```python
from build123d import *

# Parameters (mm, degrees)
BOSS_EXTRUDE1_DEPTH = 7.62
SKETCH2_R           = 1.016
BOSS_EXTRUDE2_DEPTH = 1.27


with BuildPart() as part:
    # Sketch1 → Boss-Extrude1 (new body)
    with BuildSketch(Plane(origin=(0, 0, 0), x_dir=(1, 0, 0), z_dir=(0, 1, 0))):
        Polygon((0, 1.681040649), (0, 0), (0, -1.951159351), (2.667, -1.951159351), (2.667, 1.681040649), (3.3655, 1.681040649), (3.3655, 2.935800649), (4.36372, 2.935800649), (4.36372, 5.135440649), (3.3655, 5.135440649), (3.3655, 6.583240649), (-0.6985, 6.583240649), (-0.6985, 1.681040649), align=None)
    extrude(amount=BOSS_EXTRUDE1_DEPTH)

    # Sketch2 → Boss-Extrude2 (add)
    with BuildSketch(Plane(origin=(0, 7.62, 0), x_dir=(1, 0, 0), z_dir=(0, 1, 0))):
        with Locations(Location((1.3335, 4.043240649, 0), (0, 0, 270))):
            Circle(SKETCH2_R)
    extrude(amount=BOSS_EXTRUDE2_DEPTH)


solid = part.part
```
For this review, take the finished solid that the model builds, in its own axes (mm). A direction names the side the tool comes from. Give positions to 0.01 mm unless a question says otherwise; leave off trailing zeros. Loops run counter-clockwise (first coordinate to the right, second up) from the corner with the lowest first, then second, coordinate; pieces in that order, holes last. Notation, with made-up numbers: M 21.5,89 L 51.5,89 A11 cw 51.5,105 Z; hole C 86.5,-1.5 d4. An arc over 180 degrees is marked long. One line per item, written item: value. Start each with the question number.
Q1. Add section C-C (x = 1.8). Give the boundary of the cut face in (y, z), and give its area (3 significant figures).
Q2. Clearance check with flat-ended pins moving along their axes: pin 1 Ø4 at (y, z) = (5, 1) entering from -X; pin 2 Ø0.5 at (x, y) = (4, 5.5) entering from -Z; pin 3 Ø4 at (y, z) = (3.5, 1) entering from +X. State where each tip first meets the part, or that it passes through.
Q3. For L1, parallel to X at y = 7, z = -1.25; L2, parallel to Y at x = 0, z = -3.25; L3, parallel to Z at x = 2.75, y = 6, list the stretches that pass through material, from the lowest coordinate up.
Q4. Add section A-A (y = 6). Give the boundary of the cut face in (x, z).
Q5. Add section D-D (x = 3.75). Give the boundary of the cut face in (y, z).
Q6. Machinability: for faces 1 (the face through (0, 4, 0)), 2 (the face through (4, 4, -5.135)), 3 (the face through (0.432, 8.246, -3.574)), 4 (the face through (2.667, 4, 0)), which of the approach directions +Z, -Z, +X, -X, +Y, -Y give a long, thin tool a straight path to every point of the face, cutting with its end or side? Answer none if there is none.
Q7. Add section B-B (z = -4.25). Give the boundary of the cut face in (x, y).
Reply:
1. outline: M 0,-6.58 L 7.62,-6.58 L 7.62,-4.95 L 8.89,-4.95 L 8.89,-3.14 L 7.62,-3.14 L 7.62,1.95 L 0,1.95 Z
1. area: 67.3 mm²
2. pin 1: x = 0
2. pin 2: z = -5.14
2. pin 3: x = 2.67
3. L1: 0 to 2.67
3. L2: 0 to 7.62
3. L3: -6.58 to -1.68
4. outline: M -0.7,-6.58 L 3.37,-6.58 L 3.37,-5.14 L 4.36,-5.14 L 4.36,-2.94 L 3.37,-2.94 L 3.37,-1.68 L 2.67,-1.68 L 2.67,1.95 L 0,1.95 L 0,-1.68 L -0.7,-1.68 Z
5. outline: M 0,-5.14 L 7.62,-5.14 L 7.62,-2.94 L 0,-2.94 Z
6. face 1: +Z, -X, +Y, -Y
6. face 2: -Z, +X, +Y, -Y
6. face 3: +Y
6. face 4: +Z, +X, +Y, -Y
7. outline: M -0.7,0 L 4.36,0 L 4.36,7.62 L 2.33,7.62 L 2.33,8.89 L 0.34,8.89 L 0.34,7.62 L -0.7,7.62 Z
